Geometry: final body of the model. Coordinates: model frame, mm. Give positions to 0.01 mm unless a question says otherwise; leave off trailing zeros. Write each loop counter-clockwise with the first axis right and the second up, starting at its lowest first coordinate (ties: lowest second). Pieces come first, ordered by that corner, then holes. Notation, with made-up numbers: (-31.5, 17.5) - (-11.5, 17.5) arc R7 ccw to (-11.5, 30.5) - close; hole circle Ø7 at (76, 39). An arc over 180 degrees is marked (long way). Return JSON: item names as keys, results as strings.
from build123d import *

# Parameters (mm, degrees)
SKETCH1_W                                    = 800
SKETCH1_H                                    = 800
BOSS_EXTRUDE1_DEPTH                          = 10
FILLET1_R                                    = 10
CUT_EXTRUDE1_DEPTH                           = 566.773806393
CUT_EXTRUDE1_DEPTH_BACK                      = 566.773806393
SKETCH2_R                                    = 10
SKETCH2_W                                    = 250
SKETCH2_H                                    = 200
CUT_EXTRUDE5_DEPTH                           = 566.773806393
CUT_EXTRUDE5_DEPTH_BACK                      = 566.773806393
SKETCH6_R                                    = 3
CUT_EXTRUDE6_DEPTH                           = 566.773806393
CUT_EXTRUDE6_DEPTH_BACK                      = 566.773806393
SKETCH7_R                                    = 3
CSK_FOR_M10_COUNTERSUNK_FLAT_HEAD_SC_2_COUNT = 2
CSK_FOR_M10_COUNTERSUNK_FLAT_HEAD_SC_2_PITCH = 400
CSK_FOR_M10_COUNTERSUNK_FLAT_HEAD_SC_3_COUNT = 2
CSK_FOR_M10_COUNTERSUNK_FLAT_HEAD_SC_3_PITCH = 247.487373415
CSK_FOR_M10_COUNTERSUNK_FLAT_HEAD_SC_4_COUNT = 2
CSK_FOR_M10_COUNTERSUNK_FLAT_HEAD_SC_4_PITCH = 601.040764009
CSK_FOR_M10_COUNTERSUNK_FLAT_HEAD_SC_5_COUNT = 2
CSK_FOR_M10_COUNTERSUNK_FLAT_HEAD_SC_5_PITCH = 750
CSK_FOR_M10_COUNTERSUNK_FLAT_HEAD_SC_6_COUNT = 2
CSK_FOR_M10_COUNTERSUNK_FLAT_HEAD_SC_6_PITCH = 850
CSK_FOR_M10_COUNTERSUNK_FLAT_HEAD_SC_7_COUNT = 2
CSK_FOR_M10_COUNTERSUNK_FLAT_HEAD_SC_7_PITCH = 813.172798365
CSK_FOR_M10_COUNTERSUNK_FLAT_HEAD_SC_8_COUNT = 2
CSK_FOR_M10_COUNTERSUNK_FLAT_HEAD_SC_8_PITCH = 601.040764009
M8_TAPPED_HOLE2_D                            = 6.8


with BuildPart() as part:
    # Sketch1 → Boss-Extrude1 (new body)
    with BuildSketch(Plane(origin=(0, 0, 0), x_dir=(1, 0, 0), z_dir=(0, 1, 0))):
        Rectangle(SKETCH1_W, SKETCH1_H)
    extrude(amount=BOSS_EXTRUDE1_DEPTH)

    # Fillet1
    fillet1_edges = [part.edges().sort_by_distance(p)[0] for p in [
        (400, 5, 400),
        (-400, 5, 400),
        (-400, 5, -400),
        (400, 5, -400),
    ]]
    fillet(fillet1_edges, radius=FILLET1_R)

    # Sketch2 → Cut-Extrude1 (cut, two sides: drawn at the far end of the back side and taken through both)
    with BuildSketch(Plane(origin=(0, 10, 0), x_dir=(1, 0, 0), z_dir=(0, 1, 0)).offset(-CUT_EXTRUDE1_DEPTH_BACK)):
        with Locations(Location((20, -200, 0), (0, 0, 270))):
            Circle(SKETCH2_R)
        with Locations((-225, -200)):
            Rectangle(SKETCH2_W, SKETCH2_H)
    extrude(amount=CUT_EXTRUDE1_DEPTH + CUT_EXTRUDE1_DEPTH_BACK, mode=Mode.SUBTRACT)

    # Sketch6 → Cut-Extrude5 (cut, two sides: drawn at the far end of the back side and taken through both)
    with BuildSketch(Plane(origin=(0, 10, 0), x_dir=(1, 0, 0), z_dir=(0, 1, 0)).offset(-CUT_EXTRUDE5_DEPTH_BACK)):
        with Locations(Location((-17.5, -135.048094716, 0), (0, 0, 270))):
            Circle(SKETCH6_R)
        with Locations(Location((-17.5, -264.951905284, 0), (0, 0, 270))):
            Circle(SKETCH6_R)
        with Locations(Location((95, -200, 0), (0, 0, 270))):
            Circle(SKETCH6_R)
    extrude(amount=CUT_EXTRUDE5_DEPTH + CUT_EXTRUDE5_DEPTH_BACK, mode=Mode.SUBTRACT)

    # Sketch7 → Cut-Extrude6 (cut, two sides: drawn at the far end of the back side and taken through both)
    with BuildSketch(Plane.XZ.offset(-CUT_EXTRUDE6_DEPTH_BACK)):
        with Locations(Location((-263.5, 332, 0), (0, 0, 270))):
            Circle(SKETCH7_R)
        with Locations(Location((-163.5, 332, 0), (0, 0, 270))):
            Circle(SKETCH7_R)
        with Locations(Location((-63, 255, 0), (0, 0, 270))):
            Circle(SKETCH7_R)
        with Locations(Location((-63, -145, 0), (0, 0, 270))):
            Circle(SKETCH7_R)
        with Locations(Location((-163.5, -222, 0), (0, 0, 270))):
            Circle(SKETCH7_R)
        with Locations(Location((-263.5, -222, 0), (0, 0, 270))):
            Circle(SKETCH7_R)
    extrude(amount=CUT_EXTRUDE6_DEPTH + CUT_EXTRUDE6_DEPTH_BACK, mode=Mode.SUBTRACT)

    # Sketch12 → CSK for M10 Countersunk Flat Head Screw2 (revolve, cut)
    with BuildSketch(Plane(origin=(200, 10, -375), x_dir=(0, 0, 1), z_dir=(1, 0, 0))):
        Polygon((0, 0), (0, 10), (5.5, 10), (5.5, 4.5), (10, 0), align=None)
    csk_for_m10_countersunk_flat_head_screw2 = revolve(axis=Axis((200, 16.35, -375), (0, -1, 0)), mode=Mode.SUBTRACT)

    # CSK for M10 Countersunk Flat Head Sc 2: CSK for M10 Countersunk Flat Head Screw2 ×2
    with Locations(*[(-i * CSK_FOR_M10_COUNTERSUNK_FLAT_HEAD_SC_2_PITCH, 0, 0) for i in range(1, CSK_FOR_M10_COUNTERSUNK_FLAT_HEAD_SC_2_COUNT)]):
        add(csk_for_m10_countersunk_flat_head_screw2, mode=Mode.SUBTRACT)

    # CSK for M10 Countersunk Flat Head Sc 3: CSK for M10 Countersunk Flat Head Screw2 ×2
    with Locations(*[Vector(0.7071067811865477, 0, 0.7071067811865475) * (i * CSK_FOR_M10_COUNTERSUNK_FLAT_HEAD_SC_3_PITCH) for i in range(1, CSK_FOR_M10_COUNTERSUNK_FLAT_HEAD_SC_3_COUNT)]):
        add(csk_for_m10_countersunk_flat_head_screw2, mode=Mode.SUBTRACT)

    # CSK for M10 Countersunk Flat Head Sc 4: CSK for M10 Countersunk Flat Head Screw2 ×2
    with Locations(*[Vector(0.29116161578269617, 0, 0.9566738804288585) * (i * CSK_FOR_M10_COUNTERSUNK_FLAT_HEAD_SC_4_PITCH) for i in range(1, CSK_FOR_M10_COUNTERSUNK_FLAT_HEAD_SC_4_COUNT)]):
        add(csk_for_m10_countersunk_flat_head_screw2, mode=Mode.SUBTRACT)

    # CSK for M10 Countersunk Flat Head Sc 5: CSK for M10 Countersunk Flat Head Screw2 ×2
    with Locations(*[(0, 0, i * CSK_FOR_M10_COUNTERSUNK_FLAT_HEAD_SC_5_PITCH) for i in range(1, CSK_FOR_M10_COUNTERSUNK_FLAT_HEAD_SC_5_COUNT)]):
        add(csk_for_m10_countersunk_flat_head_screw2, mode=Mode.SUBTRACT)

    # CSK for M10 Countersunk Flat Head Sc 6: CSK for M10 Countersunk Flat Head Screw2 ×2
    with Locations(*[Vector(-0.47058823529411764, 0, 0.8823529411764706) * (i * CSK_FOR_M10_COUNTERSUNK_FLAT_HEAD_SC_6_PITCH) for i in range(1, CSK_FOR_M10_COUNTERSUNK_FLAT_HEAD_SC_6_COUNT)]):
        add(csk_for_m10_countersunk_flat_head_screw2, mode=Mode.SUBTRACT)

    # CSK for M10 Countersunk Flat Head Sc 7: CSK for M10 Countersunk Flat Head Screw2 ×2
    with Locations(*[Vector(-0.7071067811865476, 0, 0.7071067811865476) * (i * CSK_FOR_M10_COUNTERSUNK_FLAT_HEAD_SC_7_PITCH) for i in range(1, CSK_FOR_M10_COUNTERSUNK_FLAT_HEAD_SC_7_COUNT)]):
        add(csk_for_m10_countersunk_flat_head_screw2, mode=Mode.SUBTRACT)

    # CSK for M10 Countersunk Flat Head Sc 8: CSK for M10 Countersunk Flat Head Screw2 ×2
    with Locations(*[Vector(-0.9566738804288585, 0, 0.291161615782696) * (i * CSK_FOR_M10_COUNTERSUNK_FLAT_HEAD_SC_8_PITCH) for i in range(1, CSK_FOR_M10_COUNTERSUNK_FLAT_HEAD_SC_8_COUNT)]):
        add(csk_for_m10_countersunk_flat_head_screw2, mode=Mode.SUBTRACT)

    # M8 Tapped Hole2 (through all)
    with Locations(Plane(origin=(0, 10, 0), x_dir=(1, 0, 0), z_dir=(0, 1, 0))):
        with Locations((180, 60), (41.435935394, 300), (318.564064606, 300)):
            Hole(M8_TAPPED_HOLE2_D / 2)


solid = part.part
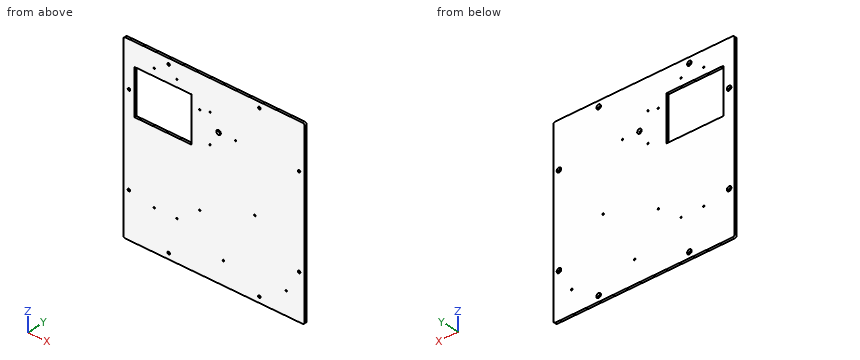
Q1. Pin query (flat end, axial travel): P1, Ø17.5, axis at x = 200, z = -375, coming from the +Y side. Return the tip coordinate at first contact, or that it passes through.
Answer key:
{"P1": "stops at y = 8.75"}
Q2. Section query A-A, the plane y = 3. Count the separate pieces of the cut face and the enclosed holes in it, plus the area to 3 significant figures.
Answer key:
{"separate pieces": "1", "enclosed holes": "22", "area": "588,000 mm^2"}
Q3. Section query B-B, the plane x = 20. Return the cut outline in (y, z), plus the area to 3 significant figures.
Answer key:
{"outline": "(0, -400) - (10, -400) - (10, 190) - (0, 190) - close; (0, 210) - (10, 210) - (10, 400) - (0, 400) - close", "area": "7,800 mm^2"}
Q4. Material intervals for probe 1 along X at (y, z) = (7, 332); probe 2 along Z at (x, y) = (198.5, 3.5); probe 3 along X at (y, z) = (3.65, -200), sorted ascending. Write a range as [from, to].
Answer key:
{"probe 1": "x = [-400, -266.5], [-260.5, -166.5], [-160.5, 400]", "probe 2": "z = [-400, -380.29], [-369.71, 369.71], [380.29, 400]", "probe 3": "x = [-400, -380.5], [-369.5, 369.5], [380.5, 400]"}
